Input: dimensioned drawing with shaded views. Units: mm. Origin: part minimum x, y, z. Round coordinates to 2 decimals unless told otherwise and drop trailing zeros. Loops run counter-clockwise (first coordinate to the right, second up) from the corner with the lowest first, then second, coordinate; pieces in that order, holes last. Notation, with made-up numbers: (14.5, -26) -> (63.5, -26) arc R34 cw to (63.5, 12) -> close; hole circle Ø7 at (42, 66). An arc over 180 degrees is marked (long way). Answer as a JSON object with one key per item and string values.
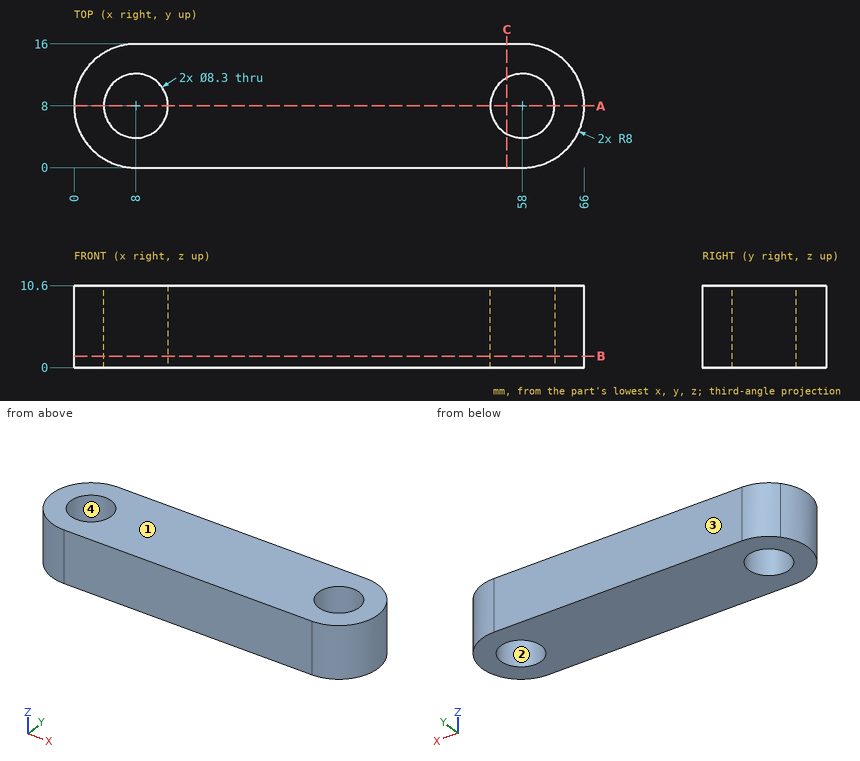
1) Ray query, probe 1 along Y at (x, z) = (8, 5.5); probe 2 along X at (y, z) = (11, 1.75); probe 3 along Y at (x, z) = (9.5, 8.25). Return the intervals inside material, ascending.
Output:
{"probe 1": "y = 0 to 3.85, 12.15 to 16", "probe 2": "x = 0.58 to 5.13, 10.87 to 55.13, 60.87 to 65.42", "probe 3": "y = 0 to 4.13, 11.87 to 16"}
2) Draft query along Y for the marked faces 1, 2, 3 and 4. Return one class per face: +Y half, -Y half, draft (parallel to the pull), parting line (faces both ways), or undercut.
Output:
{"face 1": "draft", "face 2": "undercut", "face 3": "+Y half", "face 4": "undercut"}
3) Section B-B, the plane z = 1.5. Output: boundary loops of the cut face in (x, y).
Output:
{"outline": "(8, 0) -> (58, 0) arc R8 ccw to (58, 16) -> (8, 16) arc R8 ccw to start; hole circle Ø8.3 at (8, 8); hole circle Ø8.3 at (58, 8)"}
4) Section C-C, the plane x = 56. Output: boundary loops of the cut face in (y, z), plus the area to 3 significant figures.
Output:
{"outline": "(0, 0) -> (4.36, 0) -> (4.36, 10.6) -> (0, 10.6) -> close; (11.64, 0) -> (16, 0) -> (16, 10.6) -> (11.64, 10.6) -> close", "area": "92.5 mm^2"}
5) Section A-A, the plane y = 8. Output: boundary loops of the cut face in (x, z).
Output:
{"outline": "(0, 0) -> (3.85, 0) -> (3.85, 10.6) -> (0, 10.6) -> close; (12.15, 0) -> (53.85, 0) -> (53.85, 10.6) -> (12.15, 10.6) -> close; (62.15, 0) -> (66, 0) -> (66, 10.6) -> (62.15, 10.6) -> close"}
6) Contact query for flat-ended pins moving along their axis: P1, Ø5, axis at y = 3, z = 8, coming from the -X side; P2, Ø1, axis at y = 12, z = 2, coming from the +X side. Output: stop coordinate, or through.
Output:
{"P1": "stops at x = 0.4", "P2": "stops at x = 65.19"}
